Design review of the part shown in the three views and the two pictorial views. Dimensions are in mm from the part's minimum x, y and z. Give positions to 0.01 mm unless a question says otherwise; leave off trailing zeros. Loops run counter-clockwise (first coordinate to the right, second up) from the corner with the lowest first, then second, coordinate; pieces in that order, holes last.
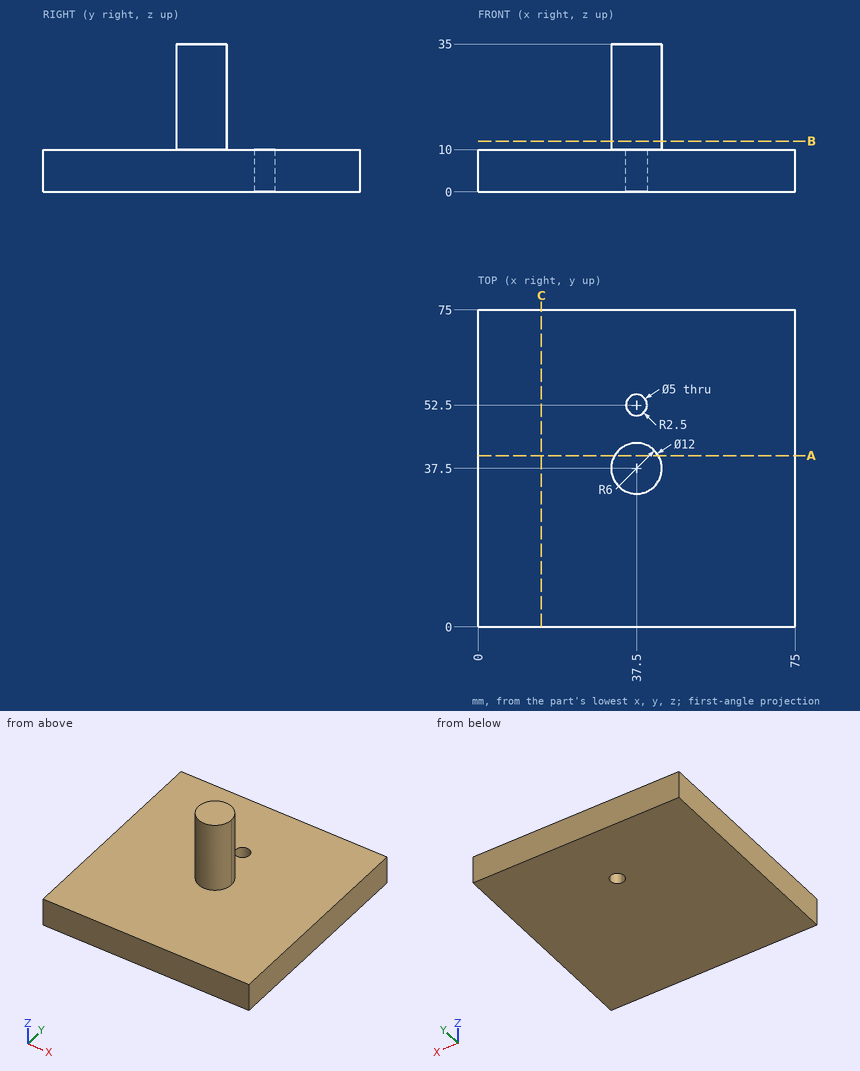
Q1. Insertion check: pin 1 (6 mm diameter, centred on x = 23.5, y = 41.5, fed in from +Z); pin 2 (6 mm diameter, centred on x = 40.5, z = 19, fed in from -Y). Each pin has a flat end and moves straight along its axis. Give the tip position at first contact, or say it passes through.
Results:
pin 1: stops at z = 10
pin 2: stops at y = 31.5
Q2. Take a section at C-C (x = 15). Give the boundary of the cut face in (y, z).
Results:
outline: (0, 0) - (75, 0) - (75, 10) - (0, 10) - close
Q3. Take a section at B-B (z = 12). Give the boundary of the cut face in (x, y).
Results:
outline: (37.5, 43.5) arc R6 ccw (long way) to (43.5, 37.5) arc R6 ccw to start
Q4. Take a section at A-A (y = 40.5). Give the boundary of the cut face in (x, z), plus the area to 3 significant figures.
Results:
outline: (0, 0) - (75, 0) - (75, 10) - (42.7, 10) - (42.7, 35) - (32.3, 35) - (32.3, 10) - (0, 10) - close
area: 1,010 mm2
Q5. Wall thickness on line 1 (Y direction, x = 37.5, z = 3); line 2 (X direction, y = 52.5, z = 7.5); line 3 (Z direction, x = 69, y = 35.5): over which ranges is each line inside the solid? List them lowest first.
Results:
line 1: y = 0 to 50, 55 to 75
line 2: x = 0 to 35, 40 to 75
line 3: z = 0 to 10
